from build123d import *

# Parameters (mm, degrees)
F0_W = 50.8
F0_H = 50.8
F4_T = -5.08


with BuildPart() as f3:
    # F0 (on Top) → F3 section 0
    with BuildSketch(Plane.XY):
        Rectangle(F0_W, F0_H)
    # F2 (on offset) → F3 section 1
    with BuildSketch(Plane.XY.offset(101.6)):
        Polygon((-0.0698438989, 35.8860855595), (-35.9559294584, -0.0698438989), (0, -35.9559294584), (35.8860855595, 0), align=None)
    loft()

    # F4
    f4_openings = [f3.faces().sort_by_distance(p)[0] for p in [
        (-0.034922, -0.034922, 101.6),
    ]]
    offset(amount=F4_T, openings=f4_openings, kind=Kind.INTERSECTION)


solid = f3.part
Can you work these out from the model? Positions are in its coordinate system, mm. Round coordinates to 2 decimals unless told otherwise and drop trailing zeros. Use one line per item in the form item = value. Start each with the question number.
Q1. We'd pull the mould along Y, two halves only. Please class faces 1 (the face through (-1, 0, 5.08)), 2 (the face through (-1, 0, 0)): +Y half, -Y half, draft (parallel to the pull), parting line (faces both ways), or undercut.
Q2. I'm going to push flat-ended pins straight in: P1, Ø1, axis at x = -10.5, y = 7.5, coming from the +Z side; P2, Ø1, axis at y = -20, z = 45.5, coming from the +X side; P3, Ø2, axis at y = 2, z = 19.5, coming from the -X side. Where does each tip first touch, or does it pass through?
Q3. If I drill on probe 1 along Z at (x, y) = (-10.5, -7); probe 2 along X at (y, z) = (-7, 6); probe 3 along X at (y, z) = (21.5, 55), over which ranges is the centre line in solid material (lowest first)? Write a range as [from, to].
Worked out:
q1.face_1 = undercut
q1.face_2 = draft
q2.P1 = 5.08
q2.P2 = 17.9
q2.P3 = -24.34
q3.probe_1 = [0, 5.08]
q3.probe_2 = [-25.31, -20.22], [19.59, 24.71]
q3.probe_3 = [-16.04, -10.42], [-2.95, 9.39]
